Geometry check sheet. Reference: the model listing, model coordinates, mm. A direction names the side the tool comes from. Give positions to 0.01 mm unless a question says otherwise; leave off trailing zeros. Write each loop counter-clockwise with the first axis right and the second up, starting at its lowest first coordinate (ties: lowest second). Pieces come first, ordered by that corner, then holes. Notation, with made-up numbers: M 60,80.25 L 113,80.25 A11 cw 113,100.25 Z; hole C 51,70.25 d3. An arc over 180 degrees is marked long. One line per item, written item: value. Start each with the question number.
1. Cross-section at D-D on y = 3.5. Count the separate pieces of the cut face and the enclosed holes in it, then the cut area to 3 significant figures.
2. Release check for a two-part mould opening along Z. For faces 6 (the face through (42, 4, -97)), 7 (the face through (-84, 4, 105)), 8 (the face through (97, 4, -42)) record: pulls with the +Z half, pulls with the -Z half, needs draft (parallel to the pull), parting line crosses it, or undercut.
3. Cross-section at B-B on x = 26. Record the cut outline in (y, z).
4. Scan lines: line 1 (X direction, y = 2.5, z = 26); line 2 (Z direction, x = -39, y = 3). Record each from-to range of solid material in increasing order.
5. Tool access check on faces 1 (the face through (-97, 4, 42)), 2 (the face through (21, 4, 101)), 3 (the face through (84, 4, 105)), 4 (the face through (21, 4, -101)), 5 (the face through (97, 4, 42)). Record the directions out of +Z, -Z, +X, -X, +Y, -Y that give a thin tool (end or side, any length) a straight path to the whole face; none if there is none.
6. Cross-section at C-C on z = -26. Record the cut outline in (x, y), then the cut area to 3 significant figures.
7. Gauge pin test, flat ends, axial feed: pin 1 (3 mm diameter, centred on y = 2.5, z = 35, fed in from -X); pin 2 (2.5 mm diameter, centred on x = 47.5, y = 2, fed in from +Z). Record the tip position at first contact, or that the pin passes through.
8. Cross-section at A-A on z = 0. Record the cut outline in (x, y).
Autodesk Inventor part; units mm, degrees
ref_plane "YZ Plane" through (0, 0, 0) normal (1, 0, 0) x (0, 1, 0)
ref_plane "XZ Plane" through (0, 0, 0) normal (0, 1, 0) x (-1, 0, 0)
ref_plane "XY Plane" through (0, 0, 0) normal (0, 0, 1) x (1, 0, 0)
sketch "Sketch2" plane through (0, 0, 0) normal (0, 1, 0) x (-1, 0, 0)
  line L0 (-105, 105) -> (105, 105)
  line L1 (105, 105) -> (105, -105)
  line L2 (105, -105) -> (-105, -105)
  line L3 (-105, -105) -> (-105, 105)
  line L4 (-105, 105) -> (105, -105) construction
  line L5 (105, 105) -> (-105, -105) construction
  circle A0 centre (0, 0) radius 10
  dimension "d11" = 210
  dimension "d12" = 210
  dimension "d13" = 20
extrude "Extrusion2" add sketch "Sketch2" along normal blind 8
sketch "Sketch3" plane through (0, 0, 0) normal (0, -1, 0) x (1, 0, 0)
  point P0 (0, 0)
  point P1 (26, 0)
  dimension "d16" = 26
hole "Hole1" at (26, 0, 0) direction (0, 1, 0) diameter 5 depth 8 tip angle 118
pattern_circular "Circular Pattern1" count 4 over 360 about axis through (0, 0, 0) along (0, 1, 0) of "Hole1"
sketch "Sketch4" plane through (0, 0, 0) normal (0, -1, 0) x (1, 0, 0)
  circle A0 centre (0, 26) radius 2.5
  circle A1 centre (-26, 0) radius 2.5
  circle A2 centre (0, -26) radius 2.5
  circle A3 centre (26, 0) radius 2.5
  circle A4 centre (0, 0) radius 10
  line L0 (105, 105) -> (-105, 105)
  line L1 (-105, 105) -> (-105, -105)
  line L2 (-105, -105) -> (105, -105)
  line L3 (105, -105) -> (105, 105)
  line L4 (-105, -63) -> (-97, -63)
  line L5 (-97, -63) -> (-97, -21)
  line L6 (-97, -21) -> (-105, -21)
  line L7 (-105, -21) -> (-105, -63)
  line L8 (-105, 21) -> (-97, 21)
  line L9 (-97, 21) -> (-97, 63)
  line L10 (-97, 63) -> (-105, 63)
  line L11 (-105, 63) -> (-105, 21)
  line L12 (-97, -21) -> (-97, 21) construction
  line L13 (-97, 63) -> (-97, 105) construction
  line L14 (-97, -63) -> (-97, -105)
  dimension "d27" = 8
extrude "Extrusion3" cut sketch "Sketch4" against normal through all contours L10 L9 L8 L1 | L4 L1 L6 L5
sketch "Sketch5" plane through (0, 0, 0) normal (0, -1, 0) x (1, 0, 0)
  line L0 (-97, 21) -> (-105, 21)
  line L1 (-105, 21) -> (-105, -21)
  line L2 (-105, -21) -> (-97, -21)
  line L3 (-97, -21) -> (-97, -63)
  line L4 (-97, -63) -> (-105, -63)
  line L5 (-105, -63) -> (-105, -105)
  line L6 (-105, -105) -> (105, -105)
  line L7 (105, -105) -> (105, 105)
  line L8 (105, 105) -> (-105, 105)
  line L9 (-105, 105) -> (-105, 63)
  line L10 (-105, 63) -> (-97, 63)
  line L11 (-97, 63) -> (-97, 21)
  circle A0 centre (0, 26) radius 2.5
  circle A1 centre (-26, 0) radius 2.5
  circle A2 centre (0, -26) radius 2.5
  circle A3 centre (26, 0) radius 2.5
  circle A4 centre (0, 0) radius 10
  line L12 (63, -105) -> (21, -105)
  line L13 (21, -105) -> (21, -97)
  line L14 (21, -97) -> (63, -97)
  line L15 (63, -97) -> (63, -105)
  line L16 (-21, -105) -> (-63, -105)
  line L17 (-63, -105) -> (-63, -97)
  line L18 (-63, -97) -> (-21, -97)
  line L19 (-21, -97) -> (-21, -105)
  line L20 (63, -97) -> (105, -97) construction
  line L21 (21, -97) -> (-21, -97) construction
  line L22 (-63, -97) -> (-105, -97) construction
  dimension "d31" = 8
extrude "Extrusion4" cut sketch "Sketch5" against normal through all contours L6 L13 L14 L15 | L17 L18 L19 L6
mirror "Mirror1" about plane through (0, 0, 0) normal (1, 0, 0) of "Extrusion3"
mirror "Mirror2" about plane through (0, 0, 0) normal (0, 0, 1) of "Extrusion4"
equation "\"d11\" = d12"
properties part number "M01 - Base Top" material "Wood (Walnut)"
Report:
1. separate pieces: 1
1. enclosed holes: 5
1. area: 41,000 mm^2
2. face 6: pulls with the -Z half
2. face 7: pulls with the +Z half
2. face 8: undercut
3. outline: M 0,-97 L 8,-97 L 8,-2.5 L 0,-2.5 Z; M 0,2.5 L 8,2.5 L 8,97 L 0,97 Z
4. line 1: x = -97 to -2.5, 2.5 to 97
4. line 2: z = -97 to 97
5. face 1: -X, +Y, -Y
5. face 2: +Z, +Y, -Y
5. face 3: +Z, +X, -X, +Y, -Y
5. face 4: -Z, +Y, -Y
5. face 5: +X, +Y, -Y
6. outline: M -97,0 L -2.5,0 L -2.5,8 L -97,8 Z; M 2.5,0 L 97,0 L 97,8 L 2.5,8 Z
6. area: 1,510 mm^2
7. pin 1: stops at x = -97
7. pin 2: stops at z = 97
8. outline: M -105,0 L -28.5,0 L -28.5,8 L -105,8 Z; M -23.5,0 L -10,0 L -10,8 L -23.5,8 Z; M 10,0 L 23.5,0 L 23.5,8 L 10,8 Z; M 28.5,0 L 105,0 L 105,8 L 28.5,8 Z
